from build123d import *

# Parameters (mm, degrees)
SKETCH_1_W           = 76
SKETCH_1_H           = 60
EXTRUDE_1_DEPTH      = 5
FILLET_1_R           = 5
SKETCH_4_R           = 1.6
CUT_EXTRUDE_3_DEPTH  = 5
SKETCH_11_R          = 10
SKETCH_11_R_2        = 1.6
CUT_EXTRUDE_11_DEPTH = 10
CUT_EXTRUDE_12_DEPTH = 13.5
FILLET_2_R           = 5
SKETCH_13_R          = 1.6
CUT_EXTRUDE_13_DEPTH = 49.672374095


with BuildPart() as part:
    # ｽｹｯﾁ1 → ﾎﾞｽ - 押し出し1 (new body)
    with BuildSketch(Plane.XY):
        Rectangle(SKETCH_1_W, SKETCH_1_H)
    extrude(amount=EXTRUDE_1_DEPTH)

    # ﾌｨﾚｯﾄ1
    fillet_1_edges = [part.edges().sort_by_distance(p)[0] for p in [
        (38, -30, 2.5),
        (-38, -30, 2.5),
        (-38, 30, 2.5),
        (38, 30, 2.5),
    ]]
    fillet(fillet_1_edges, radius=FILLET_1_R)

    # ｽｹｯﾁ4 → ｶｯﾄ - 押し出し3 (cut)
    with BuildSketch(Plane(origin=(0, 0, 0), x_dir=(-1, 0, 0), z_dir=(0, 0, -1))):
        with Locations((-33, -5)):
            Circle(SKETCH_4_R)
        with Locations((-33, -25)):
            Circle(SKETCH_4_R)
        with Locations((33, -5)):
            Circle(SKETCH_4_R)
        with Locations((33, -25)):
            Circle(SKETCH_4_R)
    extrude(amount=-CUT_EXTRUDE_3_DEPTH, mode=Mode.SUBTRACT)

    # ｽｹｯﾁ11 → ｶｯﾄ - 押し出し11 (cut)
    with BuildSketch(Plane(origin=(0, 0, 0), x_dir=(-1, 0, 0), z_dir=(0, 0, -1))):
        with Locations((0, 5)):
            Circle(SKETCH_11_R)
        with Locations((0, 18)):
            Circle(SKETCH_11_R_2)
        with Locations((13, 5)):
            Circle(SKETCH_11_R_2)
        with Locations((0, -8)):
            Circle(SKETCH_11_R_2)
        with Locations((-13, 5)):
            Circle(SKETCH_11_R_2)
    extrude(amount=-CUT_EXTRUDE_11_DEPTH, mode=Mode.SUBTRACT)

    # ｽｹｯﾁ12 → ｶｯﾄ - 押し出し12 (cut)
    with BuildSketch(Plane(origin=(0, 0, 0), x_dir=(-1, 0, 0), z_dir=(0, 0, -1))):
        with BuildLine():
            Line((-38, 0), (-20, 0))
            Line((-20, 0), (-20, 5))
            ThreePointArc((-20, 5), (0, 25), (20, 5))
            Line((20, 5), (20, 0))
            Line((20, 0), (38, 0))
            Line((38, 0), (38, 30))
            Line((38, 30), (-38, 30))
            Line((-38, 30), (-38, 0))
        make_face()
    extrude(amount=-CUT_EXTRUDE_12_DEPTH, mode=Mode.SUBTRACT)

    # ﾌｨﾚｯﾄ2
    fillet_2_edges = [part.edges().sort_by_distance(p)[0] for p in [
        (-38, 0, 2.5),
        (38, 0, 2.5),
    ]]
    fillet(fillet_2_edges, radius=FILLET_2_R)

    # ｽｹｯﾁ13 → ｶｯﾄ - 押し出し13 (cut, through all)
    with BuildSketch(Plane.XY.offset(5)):
        with Locations((16, -20)):
            Circle(SKETCH_13_R)
    extrude(amount=-CUT_EXTRUDE_13_DEPTH, mode=Mode.SUBTRACT)


solid = part.part
Here's how the part is built. I have some questions about the finished solid (model axes, mm). A direction names the side the tool comes from. Round coordinates to 2 decimals unless told otherwise and drop trailing zeros. Loops run counter-clockwise (first coordinate to the right, second up) from the corner with the lowest first, then second, coordinate; pieces in that order, holes last.
1. If we section it at C-C on x = -23: Write out the boundary of the cut face in (y, z).
Answer list:
outline: (-30, 0) - (0, 0) - (0, 5) - (-30, 5) - close
2. Which directions (+Z, -Z, +X, -X, +Y, -Y) give clear straight access to the entire face, cutting with the end or side of a thin tool? Please do faces 1 (the face through (-20, 3, 2)), 2 (the face through (-31.82, -23.92, 2.46)), 3 (the face through (20, 2, 2)).
Answer list:
face 1: +Z, -Z, -X, +Y
face 2: +Z, -Z
face 3: +Z, -Z, +X, +Y
3. We'd pull the mould along X, two halves only. Please class faces 4 (the face through (0, -30, 2)), 5 (the face through (-37, -28, 3)), 6 (the face through (-31.4, -4.93, 2.46)): +X half, -X half, draft (parallel to the pull), parting line (faces both ways), or undercut.
Answer list:
face 4: draft
face 5: -X half
face 6: undercut
4. If we section it at B-B on x = 4.5: Write out the boundary of the cut face in (y, z), plus the area to 3 significant figures.
Answer list:
outline: (-30, 0) - (-3.93, 0) - (-3.93, 5) - (-30, 5) - close; (13.93, 0) - (24.49, 0) - (24.49, 5) - (13.93, 5) - close
area: 183 mm2
5. For P1, Ø23, axis at x = 0, y = 5, coming from the +Z side; P2, Ø3, axis at x = 33, y = -5, coming from the +Z side; P3, Ø2.5, axis at x = -24.5, z = 2, coming from the +Y side; P4, Ø2.5, axis at y = 2, z = 2.5, coming from the +X side, each with a flat end and sliding along its axis, tell me the tip position at first contact or that it passes through.
Answer list:
P1: stops at z = 5
P2: passes through
P3: stops at y = 0
P4: stops at x = 20
6. If I drill on line 1 along Y through (x, z) = (33, 2.4); line 2 along Y through (x, z) = (0, 2.7); line 3 along Y through (x, z) = (-26.5, 1.05), over which ranges is the centre line in solid material (lowest first)?
Answer list:
line 1: y = -30 to -26.6, -23.4 to -6.6, -3.4 to 0
line 2: y = -30 to -9.6, -6.4 to -5, 15 to 16.4, 19.6 to 25
line 3: y = -30 to 0
7. If we section it at A-A on z = 3.2: Count the separate pieces of the cut face and the enclosed holes in it, plus the area to 3 significant figures.
Answer list:
separate pieces: 1
enclosed holes: 10
area: 2,700 mm2
